Solid Edge part; units mm, degrees
sketch "Sketch1" plane through (0, 0, 0) normal (0, -1, 0) x (1, 0, 0)
  line L0 (37.5, 20) -> (-37.5, 20)
  line L1 (-37.5, 20) -> (-37.5, 10)
  line L2 (-37.5, 10) -> (-67.5, 10)
  line L3 (-67.5, 10) -> (-67.5, 0)
  line L4 (-67.5, 0) -> (-27.5, 0)
  line L5 (-27.5, 10) -> (-27.5, 0)
  line L6 (27.5, 10) -> (-27.5, 10)
  line L7 (27.5, 0) -> (27.5, 10)
  line L8 (27.5, 0) -> (37.5, 0)
  line L9 (37.5, 0) -> (67.5, 0)
  line L10 (67.5, 0) -> (67.5, 10)
  line L11 (67.5, 10) -> (37.5, 10)
  line L12 (37.5, 10) -> (37.5, 20)
extrude "Protrusion1" add sketch "Sketch1" against normal blind 90
sketch "Sketch2" plane through (-52.5, 45, 10) normal (0, 0, 1) x (1, 0, 0)
  circle A0 centre (0, 25) radius 6
  circle A1 centre (0, -25) radius 6
  circle A2 centre (105, -25) radius 6
  circle A3 centre (105, 25) radius 6
extrude "ExtrudedCutout_1" cut sketch "Sketch2" against normal blind 48.8931
sketch "Sketch3" plane through (0, 40, 10) normal (0, -1, 0) x (1, 0, 0)
  line L0 (-67.5, 0) -> (-37.5, 10)
  line L1 (-37.5, 10) -> (-37.5, 0)
  line L2 (-37.5, 0) -> (-67.5, 0)
  line L3 (37.5, 10) -> (67.5, 0)
  line L4 (67.5, 0) -> (37.5, 0)
  line L5 (37.5, 0) -> (37.5, 10)
extrude "ExtrudedProtrusion_2" add sketch "Sketch3" along normal mid plane 3
sketch "Sketch4" plane through (37.5, 65.75, 15) normal (1, 0, 0) x (0, 1, 0)
  line L0 (-15.75, 5) -> (-15.75, 40)
  line L1 (24.25, 40) -> (24.25, 5)
  line L2 (24.25, 5) -> (-15.75, 5)
  arc A0 (-15.75, 40) -> (24.25, 40) centre (4.25, 40) cw
  circle A1 centre (4.25, 40) radius 10
extrude "ExtrudedProtrusion_3" add sketch "Sketch4" against normal blind 75
sketch "Sketch5" plane through (0, 0, 0) normal (1, 0, 0) x (0, 1, 0)
  line L0 (0, 20) -> (56.7813, 70.0089)
  line L1 (50, 55) -> (50, 20)
  line L2 (50, 20) -> (0, 20)
  arc A0 (50, 55) -> (56.7813, 70.0089) centre (70, 55) cw
extrude "ExtrudedProtrusion_4" add sketch "Sketch5" along normal mid plane 6
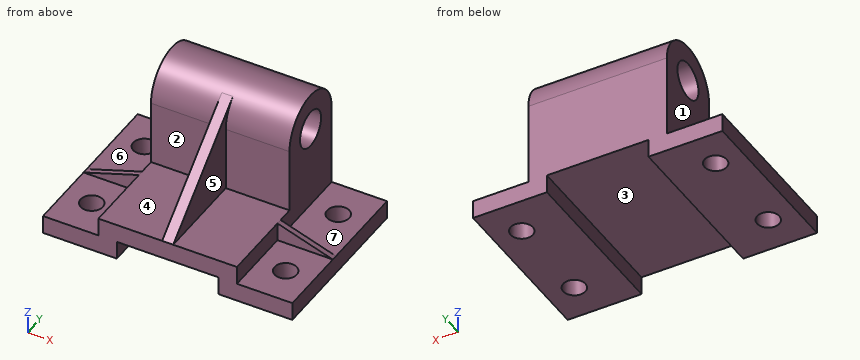
Can you work these out from the model? Positions are in its coordinate system, mm. Face numbers are marked on the shaded views. A direction names the side the tool comes from. Coordinates: 2 decimals unless noted, no trailing zeros. Write each loop counter-clockwise with the first axis right and the second up, starting at its lowest first coordinate (ties: lowest second). Pieces come first, ordered by that corner, then holes. Notation, with made-up numbers: M 59.25,35.5 L 103.25,35.5 A9 ccw 103.25,50.5 Z; hole C -37,74 d11. An arc over 180 degrees is marked long. Answer as CSV lines item,"result".
Item 1: I'm going to push flat-ended pins straight in: P1, Ø17, axis at x = 26, y = 30, coming from the +Z side; P2, Ø3, axis at y = 50.5, z = 57.5, coming from the +X side; P3, Ø24, axis at y = 74.5, z = 39, coming from the -X side; P4, Ø1.5, axis at y = 27.5, z = 47, coming from the +X side. Where does each tip first touch, or does it pass through?
Geometry results:
P1,"stops at z = 20"
P2,"stops at x = 37.5"
P3,"stops at x = -37.5"
P4,"passes through"
Item 2: On a 3-axis mill with a long thin cutter (end or side, diameter ignored), from which of +Z, -Z, +X, -X, +Y, -Y can I reach the whole of each face in a straight line? I mean the marked faces 4, 5, 6 and 7. Say none if no direction works.
Geometry results:
face 4,"+Z, -X, -Y"
face 5,"+Z, +X, -Y"
face 6,"+Z, -X, +Y"
face 7,"+Z, +X, +Y"
Item 3: We'd pull the mould along X, two halves only. Please class the marked faces 1, 2 and 3: +X half, -X half, draft (parallel to the pull), parting line (faces both ways), or undercut.
Geometry results:
face 1,"-X half"
face 2,"draft"
face 3,"undercut"
Item 4: Imagine slicing it at D-D on y = 37. List the corners of the cut face in (x, z) for me, plus the area to 3 significant figures.
Geometry results:
outline,"M -67.5,0 L -27.5,0 L -27.5,10 L 27.5,10 L 27.5,0 L 67.5,0 L 67.5,10 L 37.5,10 L 37.5,20 L 3,20 L 3,52.59 L -3,52.59 L -3,20 L -37.5,20 L -37.5,10 L -67.5,10 Z"
area,"1,750 mm2"
Item 5: Please list where these lines run through material, in increasing order: line 1 along Y through (x, z) = (-52, 6); line 2 along X through (y, z) = (69.5, 15); line 3 along Y through (x, z) = (-20, 31.5).
Geometry results:
line 1,"y = 0 to 14.02, 25.98 to 64.02, 75.98 to 90"
line 2,"x = -37.5 to 37.5"
line 3,"y = 50 to 90"
Item 6: Imagine slicing it at C-C on x = -52.5. List the corners of the cut face in (y, z) for me, plus the area to 3 significant figures.
Geometry results:
outline,"M 0,0 L 14,0 L 14,10 L 0,10 Z; M 26,0 L 64,0 L 64,10 L 41.5,10 L 41.5,15 L 38.5,15 L 38.5,10 L 26,10 Z; M 76,0 L 90,0 L 90,10 L 76,10 Z"
area,"675 mm2"
Item 7: Imagine slicing it at A-A on x = -13. List the corners of the cut face in (y, z) for me.
Geometry results:
outline,"M 0,10 L 90,10 L 90,55 A20 ccw 50,55 L 50,20 L 0,20 Z; hole C 70,55 d20"
Item 8: Imagine slicing it at B-B on y = 20. List the corners of the cut face in (x, z) for me.
Geometry results:
outline,"M -67.5,0 L -58.5,0 L -58.5,10 L -67.5,10 Z; M -46.5,0 L -27.5,0 L -27.5,10 L 27.5,10 L 27.5,0 L 46.5,0 L 46.5,10 L 37.5,10 L 37.5,20 L 3,20 L 3,37.61 L -3,37.61 L -3,20 L -37.5,20 L -37.5,10 L -46.5,10 Z; M 58.5,0 L 67.5,0 L 67.5,10 L 58.5,10 Z"
